Can you work these out from the model? Positions are in its coordinate system, mm. Face numbers are marked on the shaded views. Coordinates: 2 decimals unless noted, no trailing zeros. Loops run counter-clockwise (first coordinate to the right, second up) from the corner with the lowest first, then second, coordinate; pieces in that order, holes last. Notation, with made-up numbers: (-15.5, 67.25) - (-5.5, 67.25) arc R28 cw to (-5.5, 103.25) - close; hole circle Ø2 at (44.25, 7). An arc over 180 degrees is marked (long way). Put each result on its own line as item: value. Start each with the question number.
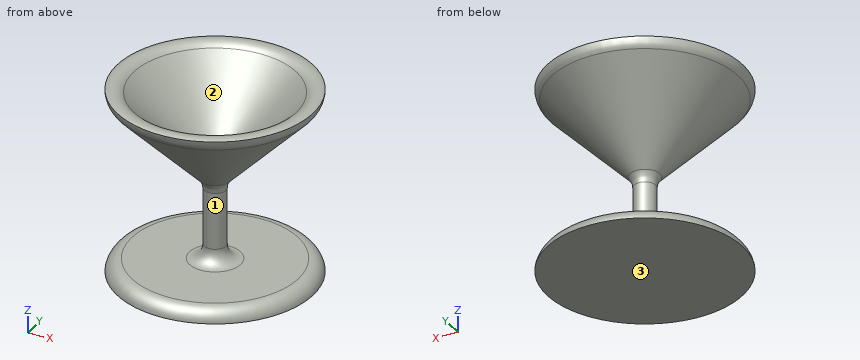
from build123d import *


# Not quite as in the source:
# - a fillet or chamfer that OpenCascade refuses, or shapes differently, is made with other operations: its cross-section is extruded or revolved along the edge and cut away or added


with BuildPart() as f1:
    # F0 (on Front) → F1 (revolve)
    with BuildSketch(Plane.XZ):
        Polygon((0, 20.1451450631), (0, 16.144845517), (2.2029185202, 18.3677908103), (19.8830971494, 36.208700271), (19.8830971494, 40.2089998171), align=None)
        Polygon((0, 2.6437440974), (0, 0), (19.8830971494, 0), (19.8830971494, 2.6437440974), (2.2029185202, 2.6437440974), align=None)
        Polygon((0, 16.144845517), (0, 2.6437440974), (2.2029185202, 2.6437440974), (2.2029185202, 18.3677908103), align=None)
    revolve(axis=Axis((0, 0, 11.3944445803), (0, 0, 1)))

    # F2: fillet of radius 3 on 3 edges, made by hand

    # F2_s1 → F2_t2 (revolve, cut)
    with BuildSketch(Plane.XZ):
        with BuildLine():
            ThreePointArc((19.8830971494, 37.4433964965), (19.6573260634, 36.3016198402), (19.0139945276, 35.331696621))
            Line((19.0139945276, 35.331696621), (19.0566124751, 35.2894626235))
            Line((19.0566124751, 35.2894626235), (19.9430971494, 36.1840063464))
            Line((19.9430971494, 36.1840063464), (19.9430971494, 37.4433964965))
            Line((19.9430971494, 37.4433964965), (19.8830971494, 37.4433964965))
        make_face()
    revolve(axis=Axis((0, 0, 36.208700271), (0, 0, 1)), mode=Mode.SUBTRACT)

    # F2_s3 → F2_t4 (revolve, cut)
    with BuildSketch(Plane.XZ):
        with BuildLine():
            ThreePointArc((19.8830971494, 0), (18.8957107839, 1.8874873657), (16.9043252998, 2.6437440974))
            Line((16.9043252998, 2.6437440974), (16.9043252998, 2.7037440974))
            Line((16.9043252998, 2.7037440974), (19.8830971494, 2.7037440974))
            Line((19.8830971494, 2.7037440974), (19.9430971494, 2.6437440974))
            ThreePointArc((19.9430971494, 2.6437440974), (19.9430971494, 1.3218720487), (19.9426725864, 0.0071251181))
            Line((19.9426725864, 0.0071251181), (19.8830971494, 0))
        make_face()
    revolve(axis=Axis((0, 0, 2.6437440974), (0, 0, 1)), mode=Mode.SUBTRACT)

    # F2_s5 → F2_t6 (revolve)
    with BuildSketch(Plane.XZ):
        with BuildLine():
            ThreePointArc((3.0720211421, 19.2447944602), (2.4286896062, 18.274871241), (2.2029185202, 17.1330945847))
            Line((2.2029185202, 17.1330945847), (2.1429185202, 17.1330945847))
            Line((2.1429185202, 17.1330945847), (2.1429185202, 18.3924847348))
            Line((2.1429185202, 18.3924847348), (3.0294031945, 19.2870284577))
            Line((3.0294031945, 19.2870284577), (3.0720211421, 19.2447944602))
        make_face()
    revolve(axis=Axis((0, 0, 18.3677908103), (0, 0, 1)))

    # F3: fillet of radius 3 on 2 edges, made by hand

    # F3_s1 → F3_t2 (revolve)
    with BuildSketch(Plane.XZ):
        with BuildLine():
            ThreePointArc((2.2029185202, 5.6437440974), (3.0815981766, 3.5224237539), (5.2029185202, 2.6437440974))
            Line((5.2029185202, 2.6437440974), (2.2029185202, 2.6437440974))
            Line((2.2029185202, 2.6437440974), (2.2029185202, 5.6437440974))
        make_face()
    revolve(axis=Axis((0, 0, 2.6437440974), (0, 0, 1)))

    # F3_s3 → F3_t4 (revolve, cut)
    with BuildSketch(Plane.XZ):
        with BuildLine():
            ThreePointArc((19.8830971494, 37.4433827054), (18.1053935902, 37.6561495071), (16.5230757584, 36.8184324094))
            Line((16.5230757584, 36.8184324094), (19.8830971494, 40.2089998171))
            Line((19.8830971494, 40.2089998171), (19.8830971494, 37.4433827054))
        make_face()
    revolve(axis=Axis((0, 0, 40.2089998171), (0, 0, 1)), mode=Mode.SUBTRACT)


solid = f1.part
Q1. I want a section at B-B on z = 18. List the corners of the cut face in (x, y) for me.
Q2. Will these pins go through, and if not, where does the flat tip stop? pin 1 (12 mm diameter, centred on x = -3, z = 33, fed in from -Y); pin 2 (5 mm diameter, centred on x = -9.5, z = 30, fed in from +Y); pin 3 (4 mm diameter, centred on x = 12.5, y = 5.5, fed in from +Z).
Q3. We'd pull the mould along Y, two halves only. Please class the marked faces 1, 2 and 3: released by +Y, released by -Y, zero draft, split by the parting line, or undercut.
Q4. Please list where these lines run through material, in increasing order: line 1 along Y through (x, z) = (-7.5, 31); line 2 along X through (y, z) = (2.5, 27.5); line 3 along Z through (x, y) = (-2, 6.5). Write a range as [from, to].
Q5. I want a section at C-C on z = 5. List the corners of the cut face in (x, y) for me, and give its area (3 significant figures).
Q6. I want a section at A-A on z = 25.5. List the corners of the cut face in (x, y) for me, and give its area (3 significant figures).
Calculated:
1. outline: circle Ø4.66 at (0, 0)
2. pin 1: y = -19.88
2. pin 2: y = 13.57
2. pin 3: z = 35.94
3. face 1: split by the parting line
3. face 2: undercut
3. face 3: zero draft
4. line 1: [-12.67, -7.71], [7.71, 12.67]
4. line 2: [-10.97, -6.85], [6.85, 10.97]
4. line 3: [0, 2.64], [23.01, 27.01]
5. outline: circle Ø4.55 at (0, 0)
5. area: 16.2 mm2
6. outline: circle Ø18.54 at (0, 0); hole circle Ø10.61 at (0, 0)
6. area: 182 mm2
